from build123d import *

# Parameters (mm, degrees)
F0_R     = 10.95
F1_DEPTH = 7


# Not quite as in the source:
# - a feature names something its author has since deleted; it is built from what else it names


with BuildPart() as f1:
    # F0 (on Top) → F1 (new body)
    with BuildSketch(Plane.XY):
        with BuildLine():
            ThreePointArc((-20.552952936, -6.752012725), (-17.9358713071, -2.6350535567), (-17.0205455745, 2.1566734649))
            ThreePointArc((-17.0205455745, 2.1566734649), (-17.6332758432, 6.1007257723), (-19.4137068981, 9.672987275))
            ThreePointArc((-19.4137068981, 9.672987275), (-33.9645978819, 14.5439431963), (-43.0205455745, 2.1566734649))
            ThreePointArc((-43.0205455745, 2.1566734649), (-36.7659143561, -8.9563819205), (-24.0205455745, -9.3758891297))
            ThreePointArc((-24.0205455745, -9.3758891297), (-22.176261837, -8.2099659445), (-20.552952936, -6.752012725))
        make_face()
        with BuildLine():
            ThreePointArc((-31.2069165924, 13.042215427), (-22.7091935329, 10.3081537797), (-19.0705455745, 2.1566734649))
            ThreePointArc((-19.0705455745, 2.1566734649), (-22.7091935329, -5.9948068499), (-31.2069165924, -8.7288684971))
            ThreePointArc((-31.2069165924, -8.7288684971), (-40.9705455745, 2.1566734649), (-31.2069165924, 13.042215427))
        make_face(mode=Mode.SUBTRACT)
        with BuildLine():
            ThreePointArc((-19.4137068981, 9.672987275), (-17.6332758432, 6.1007257723), (-17.0205455745, 2.1566734649))
            ThreePointArc((-17.0205455745, 2.1566734649), (-17.9358713071, -2.6350535567), (-20.552952936, -6.752012725))
            ThreePointArc((-20.552952936, -6.752012725), (-15.8304691356, -5.4134843039), (-11.1079853352, -6.752012725))
            ThreePointArc((-11.1079853352, -6.752012725), (-14.6092343722, 1.2571482598), (-12.2472313731, 9.672987275))
            ThreePointArc((-12.2472313731, 9.672987275), (-15.8304691356, 8.9289189085), (-19.4137068981, 9.672987275))
        make_face()
        with BuildLine():
            ThreePointArc((-24.0205455745, -9.3758891297), (-36.7659143561, -8.9563819205), (-43.0205455745, 2.1566734649))
            ThreePointArc((-43.0205455745, 2.1566734649), (-39.7569738909, -12.4615406932), (-30.0205455745, -23.8433265351))
            ThreePointArc((-30.0205455745, -23.8433265351), (-27.1231782319, -25.8236586783), (-24.0205455745, -27.4638182769))
            ThreePointArc((-24.0205455745, -27.4638182769), (-28.1334228551, -18.4198537033), (-24.0205455745, -9.3758891297))
        make_face()
        with BuildLine():
            ThreePointArc((8.9664459798, 9.672987275), (-1.6403926966, 15.1566734649), (-12.2472313731, 9.672987275))
            ThreePointArc((-12.2472313731, 9.672987275), (-14.6092343722, 1.2571482598), (-11.1079853352, -6.752012725))
            ThreePointArc((-11.1079853352, -6.752012725), (-1.6403926966, -10.8433265351), (7.8271999419, -6.752012725))
            ThreePointArc((7.8271999419, -6.752012725), (10.4442815708, -2.6350535567), (11.3596073034, 2.1566734649))
            ThreePointArc((11.3596073034, 2.1566734649), (10.7468770347, 6.1007257723), (8.9664459798, 9.672987275))
        make_face()
        with Locations((-1.6403926966, 2.1566734649)):
            Circle(F0_R, mode=Mode.SUBTRACT)
        with BuildLine():
            ThreePointArc((19.7036979596, 9.672987275), (14.3350719697, 7.8964113233), (8.9664459798, 9.672987275))
            ThreePointArc((8.9664459798, 9.672987275), (10.7468770347, 6.1007257723), (11.3596073034, 2.1566734649))
            ThreePointArc((11.3596073034, 2.1566734649), (10.4442815708, -2.6350535567), (7.8271999419, -6.752012725))
            ThreePointArc((7.8271999419, -6.752012725), (14.3350719697, -3.9687322514), (20.8429439975, -6.752012725))
            ThreePointArc((20.8429439975, -6.752012725), (17.3416949605, 1.2571482598), (19.7036979596, 9.672987275))
        make_face()
        with BuildLine():
            ThreePointArc((24.310536636, 13.6892360596), (21.767742229, 11.9556868703), (19.7036979596, 9.672987275))
            ThreePointArc((19.7036979596, 9.672987275), (17.3416949605, 1.2571482598), (20.8429439975, -6.752012725))
            ThreePointArc((20.8429439975, -6.752012725), (35.1022636576, -9.9280008025), (43.310536636, 2.1566734649))
            ThreePointArc((43.310536636, 2.1566734649), (43.2572345725, 3.0913245901), (43.1757344795, 4.0239400363))
            ThreePointArc((43.1757344795, 4.0239400363), (36.2382024635, 13.7265817549), (24.310536636, 13.6892360596))
        make_face()
        with Locations((30.310536636, 2.1566734649)):
            Circle(F0_R, mode=Mode.SUBTRACT)
        with BuildLine():
            ThreePointArc((24.310536636, 29.3296992304), (27.2086699071, 21.509467645), (24.310536636, 13.6892360596))
            ThreePointArc((24.310536636, 13.6892360596), (36.2382024635, 13.7265817549), (43.1757344795, 4.0239400363))
            ThreePointArc((43.1757344795, 4.0239400363), (39.126790521, 16.45868474), (30.310536636, 26.1173849869))
            ThreePointArc((30.310536636, 26.1173849869), (27.3989585648, 27.8886976733), (24.310536636, 29.3296992304))
        make_face()
    extrude(amount=F1_DEPTH)


solid = f1.part
Can you work these out from the model? Positions are in its coordinate system, mm. Round coordinates to 2 decimals unless told otherwise and drop trailing zeros. Loops run counter-clockwise (first coordinate to the right, second up) from the corner with the lowest first, then second, coordinate; pieces in that order, holes last. Notation, with made-up numbers: (-20, -18) - (6, -18) arc R32 ccw to (6, 8) - close; hole circle Ø8 at (33.25, 18.5). An arc over 180 degrees is marked (long way). Write item = value, one per line. Start each with the question number.
(1) If we section it at C-C (y = -2): Please give me the cut outline in (x, z), and give its area (3 significant figures).
(2) For P1, Ø1, axis at y = -1.5, z = 5.5, coming from the +X side; P2, Ø1, axis at x = -2, z = 5.5, coming from the +Y side; P3, Ø2, axis at y = -14.5, z = 5, coming from the -X side, each with a flat end and sliding along its axis, tell me the tip position at first contact or that it passes through.
(3) If we section it at A-A (x = -33): Please give me the cut outline in (y, z).
(4) If we mould it in two halves opening along Y, with no side actions, what happens to faces 1 (the face through (21.8, 11.984, 3.451)), 2 (the face through (-3, -9, 7)), 3 (the face through (19.37, 2.64, 3.45)), 4 (the face through (-22.2, -8.23, 3.45))? For each: released by +Y, released by -Y, zero draft, split by the parting line, or undercut.
(5) If we section it at B-B (z = 4.25): Please give me the cut outline in (x, y).
(6) If I drill on probe 1 along X at (y, z) = (2.5, 1.5) (3 decimals); probe 2 along X at (y, z) = (-3, 3.5); probe 3 along Y at (x, z) = (23, 5), over which ranges is the centre line in solid material (lowest first)? Write a range as [from, to].
(7) If we section it at D-D (y = 11.5): Please give me the cut outline in (x, z).
Ans:
q1.outline = (-42.84, 0) - (-40.15, 0) - (-40.15, 7) - (-42.84, 7) - close; (-19.89, 0) - (-11.77, 0) - (-11.77, 7) - (-19.89, 7) - close; (8.49, 0) - (20.18, 0) - (20.18, 7) - (8.49, 7) - close; (40.44, 0) - (42.63, 0) - (42.63, 7) - (40.44, 7) - close
q1.area = 173 mm²
q2.P1 = 42.92
q2.P2 = 15.16
q2.P3 = -39.21
q3.outline = (-21.43, 0) - (-8.38, 0) - (-8.38, 7) - (-21.43, 7) - close; (12.69, 0) - (14.81, 0) - (14.81, 7) - (12.69, 7) - close
q4.face_1 = released by +Y
q4.face_2 = zero draft
q4.face_3 = undercut
q4.face_4 = released by -Y
q5.outline = (-43.02, 2.16) arc R31 ccw to (-30.02, -23.84) arc R31 ccw to (-24.02, -27.46) arc R12 cw to (-24.02, -9.38) arc R13 ccw to (-20.55, -6.75) arc R9 cw to (-11.11, -6.75) arc R13 ccw to (7.83, -6.75) arc R9 cw to (20.84, -6.75) arc R13 ccw to (43.31, 2.16) arc R31 ccw to (30.31, 26.12) arc R31 ccw to (24.31, 29.33) arc R12 cw to (24.31, 13.69) arc R13 ccw to (19.7, 9.67) arc R9 cw to (8.97, 9.67) arc R13 ccw to (-12.25, 9.67) arc R9 cw to (-19.41, 9.67) arc R13 ccw to start; hole circle Ø21.9 at (-30.02, 2.16); hole circle Ø21.9 at (-1.64, 2.16); hole circle Ø21.9 at (30.31, 2.16)
q6.probe_1 = [-43.016, -40.965], [-19.076, -12.585], [9.304, 19.366], [41.255, 43.294]
q6.probe_2 = [-42.72, -39.68], [-20.36, -11.3], [8.02, 20.65], [39.97, 42.24]
q6.probe_3 = [-8.59, -6], [10.31, 12.91]
q7.outline = (-39.06, 0) - (-35.73, 0) - (-35.73, 7) - (-39.06, 7) - close; (-24.31, 0) - (-20.98, 0) - (-20.98, 7) - (-24.31, 7) - close; (-10.68, 0) - (-7.35, 0) - (-7.35, 7) - (-10.68, 7) - close; (4.07, 0) - (7.4, 0) - (7.4, 7) - (4.07, 7) - close; (21.27, 0) - (24.6, 0) - (24.6, 7) - (21.27, 7) - close; (36.02, 0) - (41.45, 0) - (41.45, 7) - (36.02, 7) - close
